Verification items for this drawing (mm, ordinates from the low corner). A direction names the side the tool comes from. Round coordinates to 2 decimals unless told otherwise and drop trailing zeros. Loops run counter-clockwise (first coordinate to the right, second up) from the corner with the lowest first, then second, coordinate; pieces in that order, holes last. Notation, with made-up numbers: M 73,46.5 L 95,46.5 A17 ccw 95,58.5 Z; hole C 13,86 d3. An arc over 180 degrees is marked long. Use one line per item in the form item = value. Start each with the question number.
1. Go/stop test with flat-tipped pins: pin 1 (1.5 mm diameter, centred on x = 63, z = 8, fed in from -Y); pin 2 (1.5 mm diameter, centred on y = 17.5, z = 14, fed in from +X); pin 3 (7 mm diameter, centred on x = 130, z = 12, fed in from -Y); pin 4 (5 mm diameter, centred on x = 132, z = 16, fed in from +Y). Record where each tip stops, or that it passes through.
2. Cross-section at D-D (x = 105). Record the boundary of the cut face in (y, z).
3. Cross-section at B-B (z = 10.25). Record the boundary of the cut face in (x, y) (1 decimal).
4. Cross-section at A-A (y = 3). Record the boundary of the cut face in (x, z), then the cut area to 3 significant figures.
5. Set-up check for the marked faces 4, 5 and 6: record each of +Z, -Z, +X, -X, +Y, -Y from which the full face is reachable in a straight line by a thin tool's end or side.
6. Material ranges on line 1 (X direction, y = 8.5, z = 21); line 2 (Z direction, x = 130, y = 25.5); line 3 (X direction, y = 21.75, z = 12), recorded low to high.
7. Cross-section at C-C (x = 130). Record the boundary of the cut face in (y, z), then the cut area to 3 significant figures.
8. Draft check along X on the marked faces 1, 2 and 3. Enter one of: pulls with the +X half, pulls with the -X half, needs draft (parallel to the pull), parting line crosses it, or undercut.
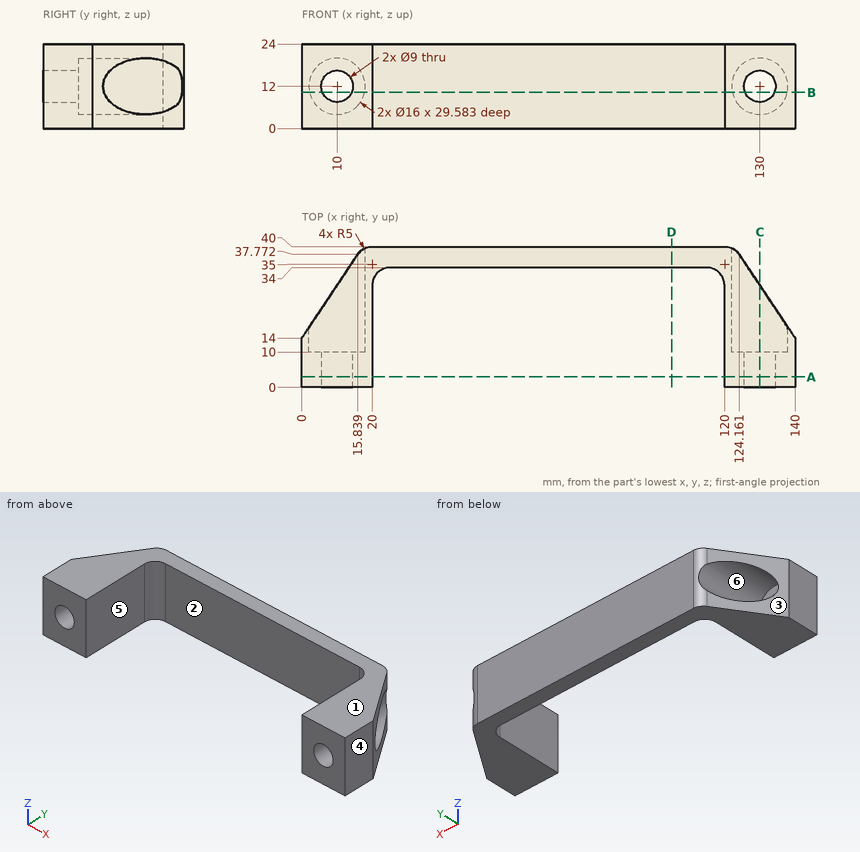
Reported:
q1.pin_1 = 34
q1.pin_2 = 138.17
q1.pin_3 = through
q1.pin_4 = 10
q2.outline = M 34,0 L 40,0 L 40,24 L 34,24 Z
q3.outline = M 0,0 L 5.9,0 L 5.9,10 L 2.2,10 L 2.2,17.3 L 0,14 Z; M 14.1,0 L 20,0 L 20,29 A5 cw 25,34 L 115,34 A5 cw 120,29 L 120,0 L 125.9,0 L 125.9,10 L 122.2,10 L 122.2,39.5 A5 ccw 120,40 L 20,40 A5 ccw 17.8,39.5 L 17.8,10 L 14.1,10 Z; M 134.1,0 L 140,0 L 140,14 L 137.8,17.3 L 137.8,10 L 134.1,10 Z
q4.outline = M 0,0 L 20,0 L 20,24 L 0,24 Z; M 120,0 L 140,0 L 140,24 L 120,24 Z; hole C 10,12 d9; hole C 130,12 d9
q4.area = 833 mm²
q5.face_4 = +Z, -Z, +X, +Y, -Y
q5.face_5 = +Z, -Z, -Y
q5.face_6 = +Y
q6.line_1 = 0 to 20, 120 to 140
q6.line_2 = 0 to 4, 20 to 24
q6.line_3 = 18 to 20, 120 to 122
q7.outline = M 0,0 L 29.01,0 L 29.01,4 L 10,4 L 10,7.5 L 0,7.5 Z; M 0,16.5 L 10,16.5 L 10,20 L 29.01,20 L 29.01,24 L 0,24 Z
q7.area = 302 mm²
q8.face_1 = needs draft
q8.face_2 = undercut
q8.face_3 = pulls with the -X half
